Could you check a few things on this model? Use its own coordinates, in mm. Coordinates: 2 decimals unless noted, no trailing zeros. Write each loop counter-clockwise with the first axis right and the second up, starting at its lowest first coordinate (ties: lowest second). Pieces come first, ordered by that corner, then holes.
```python
from build123d import *

# Parameters (mm, degrees)
BOSS_EXTRUDE1_DEPTH = 0.254
SKETCH2_R           = 4.699
CUT_EXTRUDE1_DEPTH  = 1.254
SKETCH3_W           = 2.54
SKETCH3_H           = 0.635
CUT_EXTRUDE2_DEPTH  = 1.254
CUT_EXTRUDE3_DEPTH  = 1.254


with BuildPart() as part:
    # Sketch1 → Boss-Extrude1 (new body)
    with BuildSketch(Plane.XY):
        with BuildLine():
            Line((27.218819563, 62.393373411), (22.357699804, 50.65759216))
            ThreePointArc((22.357699804, 50.65759216), (28.61353693, 47.405947816), (34.405475059, 43.38573118))
            Line((34.405475059, 43.38573118), (8.696654013, 17.676910134))
            Line((8.696654013, 17.676910134), (7.228954972, 14.133571205))
            ThreePointArc((7.228954972, 14.133571205), (14.666587579, 6.075099489), (15.105587123, -4.88230096))
            Line((15.105587123, -4.88230096), (18.648926052, -6.35))
            Line((18.648926052, -6.35), (101.401368334, -6.35))
            ThreePointArc((101.401368334, -6.35), (93.866160503, 38.880636728), (67.21146711, 76.191723231))
            Line((67.21146711, 76.191723231), (43.43415954, 52.414415661))
            ThreePointArc((43.43415954, 52.414415661), (35.677104191, 57.973626939), (27.218819563, 62.393373411))
        make_face()
        with BuildLine():
            Line((88.672924278, 6.35), (27.86051193, 6.35))
            ThreePointArc((27.86051193, 6.35), (26.399857642, 10.93517908), (24.190484974, 15.210228852))
            Line((24.190484974, 15.210228852), (67.191354125, 58.211098004))
            ThreePointArc((67.191354125, 58.211098004), (82.13289044, 34.020557137), (88.672924278, 6.35))
        make_face(mode=Mode.SUBTRACT)
    extrude(amount=BOSS_EXTRUDE1_DEPTH)

    # Sketch2 → Cut-Extrude1 (cut, through all)
    with BuildSketch(Plane.XY.offset(0.254)):
        with Locations((22.225, 0)):
            Circle(SKETCH2_R)
        with Locations((36.195, 0)):
            Circle(SKETCH2_R)
        with Locations((61.722, 0)):
            Circle(SKETCH2_R)
        with Locations((75.692, 0)):
            Circle(SKETCH2_R)
        with Locations((95.25, 0)):
            Circle(SKETCH2_R)
        with Locations((15.715448212, 15.715448212)):
            Circle(SKETCH2_R)
        with Locations((25.593729945, 25.593729945)):
            Circle(SKETCH2_R)
        with Locations((43.644044748, 43.644044748)):
            Circle(SKETCH2_R)
        with Locations((53.522326482, 53.522326482)):
            Circle(SKETCH2_R)
        with Locations((92.004434954, 24.652514046)):
            Circle(SKETCH2_R)
        with Locations((82.48891971, 47.625)):
            Circle(SKETCH2_R)
        with Locations((67.351920908, 67.351920908)):
            Circle(SKETCH2_R)
        with Locations((30.861, 53.452819972)):
            Circle(SKETCH2_R)
    extrude(amount=-CUT_EXTRUDE1_DEPTH, mode=Mode.SUBTRACT)

    # Sketch3 → Cut-Extrude2 (cut, through all)
    with BuildSketch(Plane.XY.offset(0.254)):
        Polygon((15.266435406, 24.246691527), (17.06248663, 26.042742751), (17.511499436, 25.593729945), (15.715448212, 23.797678721), align=None)
        Polygon((43.43415954, 52.414415661), (44.991083167, 53.971339288), (45.440095973, 53.522326482), (43.883172346, 51.965402855), align=None)
        with Locations((29.21, -6.0325)):
            Rectangle(SKETCH3_W, SKETCH3_H)
        with Locations((68.707, -6.0325)):
            Rectangle(SKETCH3_W, SKETCH3_H)
        Polygon((29.230733674, 38.210989795), (31.026784898, 40.007041019), (31.475797704, 39.558028213), (29.67974648, 37.761976989), align=None)
        Polygon((56.845021246, 65.825277367), (55.048970022, 64.029226143), (55.497982828, 63.580213337), (57.294034052, 65.376264561), align=None)
        with Locations((48.9585, -6.0325)):
            Rectangle(SKETCH3_W, SKETCH3_H)
        with Locations((85.471, -6.0325)):
            Rectangle(SKETCH3_W, SKETCH3_H)
        Polygon((99.935462164, 14.437711971), (100.266998693, 11.919442024), (101.526133667, 12.085210288), (101.194597138, 14.603480236), align=None)
        Polygon((93.765504959, 37.464305742), (94.938831965, 37.950313702), (93.966816047, 40.296967714), (92.793489041, 39.810959755), align=None)
        Polygon((79.327792988, 62.471156422), (80.874047017, 60.456038938), (81.88160576, 61.229165953), (80.33535173, 63.244283437), align=None)
        Polygon((13.593916116, 7.005422516), (14.565932035, 4.658768503), (15.739259041, 5.144776462), (14.767243123, 7.491430475), align=None)
    extrude(amount=-CUT_EXTRUDE2_DEPTH, mode=Mode.SUBTRACT)

    # Sketch7 → Cut-Extrude3 (cut, through all)
    with BuildSketch(Plane.XY.offset(0.254)):
        with BuildLine():
            Line((36.195, 4.699), (61.722, 4.699))
            ThreePointArc((61.722, 4.699), (66.421, 0), (61.722, -4.699))
            Line((61.722, -4.699), (36.195, -4.699))
            ThreePointArc((36.195, -4.699), (31.496, 0), (36.195, 4.699))
        make_face()
        with BuildLine():
            Line((75.692, 4.699), (95.25, 4.699))
            ThreePointArc((95.25, 4.699), (99.949, 0), (95.25, -4.699))
            Line((95.25, -4.699), (75.692, -4.699))
            ThreePointArc((75.692, -4.699), (70.993, 0), (75.692, 4.699))
        make_face()
        with BuildLine():
            Line((50.199631717, 56.845021246), (64.029226143, 70.674615673))
            ThreePointArc((64.029226143, 70.674615673), (70.674615673, 70.674615673), (70.674615673, 64.029226143))
            Line((70.674615673, 64.029226143), (56.845021246, 50.199631717))
            ThreePointArc((56.845021246, 50.199631717), (50.199631717, 50.199631717), (50.199631717, 56.845021246))
        make_face()
        with BuildLine():
            ThreePointArc((46.966739513, 46.966739513), (40.434542876, 52.695322215), (33.2105, 57.522273345))
            ThreePointArc((33.2105, 57.522273345), (26.791546628, 55.802319972), (28.5115, 49.3833666))
            ThreePointArc((28.5115, 49.3833666), (34.713402966, 45.239387523), (40.321349984, 40.321349984))
            ThreePointArc((40.321349984, 40.321349984), (46.966739513, 40.321349984), (46.966739513, 46.966739513))
        make_face()
        with BuildLine():
            ThreePointArc((26.924, 0), (24.874532533, 10.303368733), (19.038142977, 19.038142977))
            ThreePointArc((19.038142977, 19.038142977), (12.392753447, 19.038142977), (12.392753447, 12.392753447))
            ThreePointArc((12.392753447, 12.392753447), (16.191912687, 6.706909836), (17.526, 0))
            ThreePointArc((17.526, 0), (22.225, -4.699), (26.924, 0))
        make_face()
        with BuildLine():
            ThreePointArc((96.543320412, 25.868704739), (92.340835395, 38.248826381), (86.558373083, 49.9745))
            ThreePointArc((86.558373083, 49.9745), (80.13941971, 51.694453372), (78.419466338, 45.2755))
            ThreePointArc((78.419466338, 45.2755), (83.658215548, 34.652367484), (87.465549496, 23.436323353))
            ThreePointArc((87.465549496, 23.436323353), (93.220625647, 20.113628588), (96.543320412, 25.868704739))
        make_face()
    extrude(amount=-CUT_EXTRUDE3_DEPTH, mode=Mode.SUBTRACT)


solid = part.part
```
1. I want a section at B-B on z = 0.1. Give the number of separate pieces and of enclosed holes in the cut face, plus the area to 3 significant figures.
Verdict:
separate pieces: 1
enclosed holes: 8
area: 1,580 mm2
2. Please list where these lines run through material, in increasing order: line 1 along X through (y, z) = (14, 0.1); line 2 along X through (y, z) = (-3, 0.2); line 3 along Y through (x, z) = (65.5, 0.15).
Verdict:
line 1: x = 7.48 to 11.34, 23 to 24.91, 87.79 to 99.99
line 2: x = 15.59 to 18.61, 25.84 to 32.58, 65.34 to 72.08, 98.87 to 101.56
line 3: y = -6.35 to -2.79, 2.79 to 6.35, 56.52 to 58.85, 71.67 to 74.48
3. For pin 1 (7.5 mm diameter, centred on x = 25.59, y = 25.59, fed in from -Z), with a flat end and sliding along its axis, tell me the tip position at first contact or that it passes through.
Verdict:
pin 1: passes through
4. I want a section at A-A on y = 16.5. Please give me the cut outline in (x, z), plus the area to 3 significant figures.
Verdict:
outline: (8.21, 0) - (11.08, 0) - (11.08, 0.25) - (8.21, 0.25) - close; (21.28, 0) - (25.48, 0) - (25.48, 0.25) - (21.28, 0.25) - close; (87.36, 0) - (100.25, 0) - (100.25, 0.25) - (87.36, 0.25) - close
area: 5.07 mm2
